The model under review builds one solid part; all positions refer to its coordinate system, in mm. A direction names the side the tool comes from. Coordinates: 2 decimals unless noted, no trailing zeros. Order: outer loops, then holes, each group sorted by start corner. A loop starts at its lowest first (then second) coordinate and runs counter-clockwise, first axis right, second up.
from build123d import *

# Parameters (mm, degrees)
SKETCH1_W                = 80
SKETCH1_H                = 140
BOSS_EXTRUDE1_DEPTH      = 25
BOSS_EXTRUDE2_DEPTH      = 30
BOSS_EXTRUDE2_DEPTH_BACK = 30
BOSS_EXTRUDE3_REACH      = 135.781
SKETCH3_R                = 15
SKETCH3_R_2              = 10
BOSS_EXTRUDE7_DEPTH      = 30
BOSS_EXTRUDE8_DEPTH      = 20
CUT_EXTRUDE1_REACH       = 202.087


with BuildPart() as part:
    # Sketch1 → Boss-Extrude1 (new body)
    with BuildSketch(Plane(origin=(0, 0, 0), x_dir=(1, 0, 0), z_dir=(0, 1, 0))):
        with Locations((3.446067736, -28.029835879)):
            Rectangle(SKETCH1_W, SKETCH1_H)
    extrude(amount=BOSS_EXTRUDE1_DEPTH)

    # Sketch2 → Boss-Extrude2 (add, two sides: drawn at the far end of the back side and taken through both)
    with BuildSketch(Plane(origin=(0, 0, 0), x_dir=(0, 0, -1), z_dir=(1, 0, 0)).offset(-BOSS_EXTRUDE2_DEPTH_BACK)):
        with BuildLine():
            Line((31.970164121, 25), (31.970164121, 135))
            Line((31.970164121, 135), (1.970164121, 135))
            Line((1.970164121, 135), (1.970164121, 95))
            ThreePointArc((1.970164121, 95), (-18.532361196, 45.502525317), (-68.029835879, 25))
            Line((-68.029835879, 25), (31.970164121, 25))
        make_face()
    extrude(amount=BOSS_EXTRUDE2_DEPTH + BOSS_EXTRUDE2_DEPTH_BACK)

    # Sketch3 → Boss-Extrude3 (add, up to next)
    with BuildSketch(Plane(origin=(0, 55, 0), x_dir=(1, 0, 0), z_dir=(0, 1, 0)), mode=Mode.PRIVATE) as boss_extrude3_sk1:
        with Locations(Location((0, -73.029835879, 0), (0, 0, 270))):
            Circle(SKETCH3_R)
        with Locations(Location((0, -73.029835879, 0), (0, 0, 270))):
            Circle(SKETCH3_R_2, mode=Mode.SUBTRACT)
    boss_extrude3_tool1 = extrude(boss_extrude3_sk1.sketch, amount=-BOSS_EXTRUDE3_REACH, mode=Mode.PRIVATE) - part.part
    add(boss_extrude3_tool1.solids().sort_by_distance((0, 55, 58.4541))[0])

    # Sketch4 → Boss-Extrude7 (add)
    with BuildSketch(Plane(origin=(0, 50, 0), x_dir=(1, 0, 0), z_dir=(0, 1, 0))):
        with BuildLine():
            ThreePointArc((-15, -73.029835859), (6e-09, -58.029835879), (15, -73.029835871))
            Line((15, -73.029835871), (15, -7.547322413))
            Line((15, -7.547322413), (-15, -7.547322413))
            Line((-15, -7.547322413), (-15, -73.029835859))
        make_face()
    extrude(amount=-BOSS_EXTRUDE7_DEPTH)

    # Sketch7 → Boss-Extrude8 (add)
    with BuildSketch(Plane(origin=(0, 135, 0), x_dir=(1, 0, 0), z_dir=(0, 1, 0))):
        with BuildLine():
            Line((12.629019998, -36.512692343), (12.629019998, -68.029835879))
            Line((12.629019998, -68.029835879), (-12.629019998, -68.029835879))
            Line((-12.629019998, -68.029835879), (-12.629019998, -36.512692343))
            ThreePointArc((-12.629019998, -36.512692343), (-23.188563942, -22.185014582), (-40, -28.029835879))
            Line((-40, -28.029835879), (-40, 39.970164121))
            Line((-40, 39.970164121), (40, 39.970164121))
            Line((40, 39.970164121), (40, -28.029835879))
            ThreePointArc((40, -28.029835879), (23.188563942, -22.185014582), (12.629019998, -36.512692343))
        make_face()
    extrude(amount=BOSS_EXTRUDE8_DEPTH)

    # Sketch8 → Cut-Extrude1 (cut, up to next)
    with BuildSketch(Plane(origin=(40, 0, 0), x_dir=(0, 0, -1), z_dir=(1, 0, 0)), mode=Mode.PRIVATE) as cut_extrude1_sk1:
        Polygon((21.970164121, 155), (39.970164121, 155), (39.970164121, 150), align=None)
    cut_extrude1_tool1 = extrude(cut_extrude1_sk1.sketch, amount=-CUT_EXTRUDE1_REACH, mode=Mode.PRIVATE) & part.part
    # Sketch8 → Cut-Extrude1 (cut, up to next)
    with BuildSketch(Plane(origin=(40, 0, 0), x_dir=(0, 0, -1), z_dir=(1, 0, 0)), mode=Mode.PRIVATE) as cut_extrude1_sk2:
        with BuildLine():
            Line((-13.029835879, 155), (6.970164121, 155))
            ThreePointArc((6.970164121, 155), (-3.029835879, 145), (-13.029835879, 155))
        make_face()
    cut_extrude1_tool2 = extrude(cut_extrude1_sk2.sketch, amount=-CUT_EXTRUDE1_REACH, mode=Mode.PRIVATE) & part.part
    add(cut_extrude1_tool1.solids().sort_by_distance((40, 153.333333, -33.970164))[0], mode=Mode.SUBTRACT)
    add(cut_extrude1_tool2.solids().sort_by_distance((40, 150.755868, 3.029836))[0], mode=Mode.SUBTRACT)


solid = part.part
(1) Insertion check: pin 1 Ø10 at (x, y) = (2, 149) entering from +Z; pin 2 Ø16.5 at (x, z) = (-0.5, 73) entering from +Y; pin 3 Ø1.5 at (x, y) = (13.5, 48.5) entering from -Z; pin 4 Ø10 at (y, z) = (149.5, -14.5) entering from +X. Each pin has a flat end and moves straight along its axis. Give the tip position at first contact, or say it passes through.
(2) Consider section B-B (z = 25). Give the boundary of the cut face in (x, y).
(3) Consider section A-A (x = 33). Give the boundary of the cut face in (y, z), then the cut area to 3 significant figures.
(4) Wall thickness on line 1 (Y direction, x = 35, z = -10); line 2 (Z direction, x = 0, y = 45.5); line 3 (X direction, y = 34, z = 11): over which ranges is each line inside the solid? List them lowest first.
(5) Consider section D-D (z = 9). Give the boundary of the cut face in (x, y), then the cut area to 3 significant figures.
(6) The part is to be moulded in two halves that separate along Y. For faces 1 (the face through (3, 0, 27)), 2 (the face through (38, 25, 27)), 3 (the face through (-36.554, 12, 29)), say which applies: +Y half, -Y half, draft (parallel to the pull), parting line (faces both ways), or undercut.
(7) Consider section C-C (x = 0). Give the boundary of the cut face in (y, z), then the cut area to 3 significant figures.
(8) Tool access review of faces 4 (the face through (23.44, 144.86, 22.11)), 5 (the face through (-30, 69, -15)), 6 (the face through (30, 69, -15)), 7 (the face through (-0.12, 25.03, 66.05)), 8 (the face through (-3, 55, 83)): name each direction out of +Z, -Z, +X, -X, +Y, -Y from which nothing blocks a thin tool from reaching the whole face with its end or side.
Findings:
1. pin 1: stops at z = 68.03
1. pin 2: stops at y = 155
1. pin 3: stops at z = -31.97
1. pin 4: stops at x = 40
2. outline: (-40, 135) - (-37.24, 135) - (-37.24, 155) - (-40, 155) - close; (-36.55, 0) - (43.45, 0) - (43.45, 25) - (30, 25) - (30, 39.79) - (15, 39.79) - (15, 50) - (-15, 50) - (-15, 39.79) - (-30, 39.79) - (-30, 25) - (-36.55, 25) - close; (-18.01, 135) - (18.01, 135) - (18.01, 155) - (-18.01, 155) - close; (37.24, 135) - (40, 135) - (40, 155) - (37.24, 155) - close
3. outline: (0, -41.97) - (25, -41.97) - (25, 98.03) - (0, 98.03) - close; (135, -39.97) - (150, -39.97) - (155, -21.97) - (155, -6.97) arc R10 cw to (155, 13.03) - (155, 22.51) - (135, 22.51) - close
3. area: 4,550 mm2
4. line 1: y = 0 to 25, 135 to 155
4. line 2: z = -31.97 to 63.03, 83.03 to 88.03
4. line 3: x = -30 to 30
5. outline: (-40, 135) - (40, 135) - (40, 146.98) - (-40, 146.98) - close; (-36.55, 0) - (43.45, 0) - (43.45, 25) - (30, 25) - (30, 57.38) - (-30, 57.38) - (-30, 25) - (-36.55, 25) - close
5. area: 4,900 mm2
6. face 1: -Y half
6. face 2: undercut
6. face 3: draft
7. outline: (0, -41.97) - (25, -41.97) - (25, -31.97) - (135, -31.97) - (135, -39.97) - (150, -39.97) - (155, -21.97) - (155, -6.97) arc R10 cw to (155, 13.03) - (155, 68.03) - (135, 68.03) - (135, -1.97) - (95, -1.97) arc R70 cw to (50, 14.41) - (50, 58.03) - (55, 58.03) - (55, 63.03) - (25.18, 63.03) arc R70 cw to (25, 68.03) - (25, 83.03) - (55, 83.03) - (55, 88.03) - (25, 88.03) - (25, 98.03) - (0, 98.03) - close
7. area: 10,800 mm2
8. face 4: +Z, +Y
8. face 5: +Z, -Z, -X
8. face 6: +Z, -Z, +X
8. face 7: none
8. face 8: +Z, +X, -X
